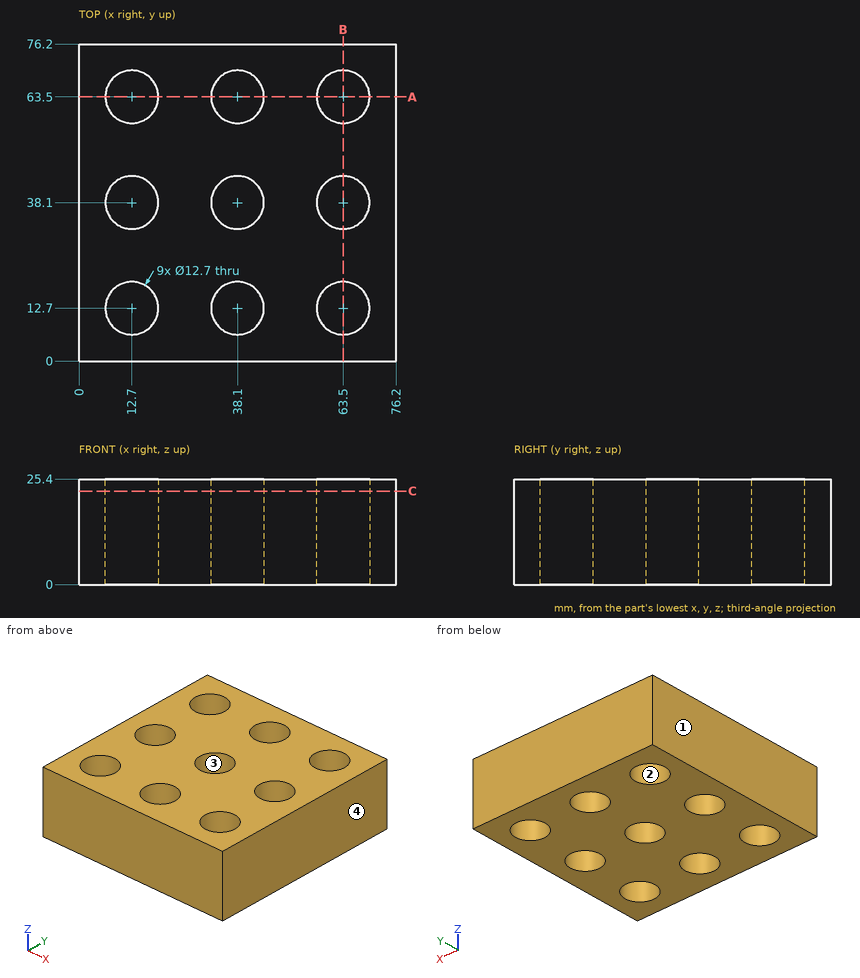
Design review of the part shown in the three views and the two pictorial views. Dimensions are in mm from the part's minimum x, y and z. Round coordinates to 2 decimals unless told otherwise and drop trailing zeros. Loops run counter-clockwise (first coordinate to the right, second up) from the corner with the lowest first, then second, coordinate; pieces in that order, holes last.
1) Consider section C-C on z = 22.5. Give the number of separate pieces and of enclosed holes in the cut face, then the cut area to 3 significant figures.
Values follow:
separate pieces: 1
enclosed holes: 9
area: 4,670 mm2
2) Wall thickness on line 1 along Y through (x, z) = (12.7, 18.75); line 2 along Y through (x, z) = (61.5, 9.25); line 3 along X through (y, z) = (11, 20.5): over which ranges is each line inside the solid? List them lowest first.
Values follow:
line 1: y = 0 to 6.35, 19.05 to 31.75, 44.45 to 57.15, 69.85 to 76.2
line 2: y = 0 to 6.67, 18.73 to 32.07, 44.13 to 57.47, 69.53 to 76.2
line 3: x = 0 to 6.58, 18.82 to 31.98, 44.22 to 57.38, 69.62 to 76.2
3) The part is to be moulded in two halves that separate along X. For the marked faces 1, 2, 3 and 4, say which applies: pulls with the +X half, pulls with the -X half, needs draft (parallel to the pull), parting line crosses it, or undercut.
Values follow:
face 1: pulls with the -X half
face 2: undercut
face 3: undercut
face 4: pulls with the +X half
4) Consider section A-A on y = 63.5. State the section outline as (x, z) points, then the cut area to 3 significant figures.
Values follow:
outline: (0, 0) - (6.35, 0) - (6.35, 25.4) - (0, 25.4) - close; (19.05, 0) - (31.75, 0) - (31.75, 25.4) - (19.05, 25.4) - close; (44.45, 0) - (57.15, 0) - (57.15, 25.4) - (44.45, 25.4) - close; (69.85, 0) - (76.2, 0) - (76.2, 25.4) - (69.85, 25.4) - close
area: 968 mm2
